The model under review builds one solid part; all positions refer to its coordinate system, in mm. A direction names the side the tool comes from. Coordinates: 2 decimals unless noted, no trailing zeros. Write each loop counter-clockwise with the first axis right and the second up, starting at its lowest first coordinate (ties: lowest second). Pieces come first, ordered by that corner, then holes. Notation, with made-up numbers: M 30.5,73 L 47.5,73 A24 cw 47.5,95 Z; hole C 34.5,17.5 d10. An arc over 180 degrees is marked long. Answer as CSV lines item,"result". Start each with the question number.
from build123d import *

# Parameters (mm, degrees)
BOSS_EXTRUDE1_DEPTH = 42
FILLET1_R           = 3
SKETCH3_R           = 4.25
CUT_EXTRUDE1_DEPTH  = 50.500549163
BOSS_EXTRUDE2_DEPTH = 42
CUT_EXTRUDE2_DEPTH  = 50.678098566


with BuildPart() as part:
    # Sketch1 → Boss-Extrude1 (new body)
    with BuildSketch(Plane(origin=(0, 0, 0), x_dir=(1, 0, 0), z_dir=(0, 1, 0))):
        with BuildLine():
            Line((-7.705313318, 23.08749092), (1.86118947, 26))
            ThreePointArc((1.86118947, 26), (5.698552556, 0), (1.86118947, -26))
            Line((1.86118947, -26), (-7.705313318, -23.08749092))
            ThreePointArc((-7.705313318, -23.08749092), (-4.301447444, 0), (-7.705313318, 23.08749092))
        make_face()
    extrude(amount=BOSS_EXTRUDE1_DEPTH)

    # Fillet1
    fillet1_edges = [part.edges().sort_by_distance(p)[0] for p in [
        (-7.705313318, 21, -23.08749092),
        (1.86118947, 21, -26),
        (1.86118947, 21, 26),
        (-7.705313318, 21, 23.08749092),
    ]]
    fillet(fillet1_edges, radius=FILLET1_R)

    # Sketch3 → Cut-Extrude1 (cut, through all)
    with BuildSketch(Plane(origin=(0, 42, 0), x_dir=(1, 0, 0), z_dir=(0, 1, 0))):
        with Locations(Location((0.733117745, 0, 0), (0, 0, 270))):
            Circle(SKETCH3_R)
    extrude(amount=-CUT_EXTRUDE1_DEPTH, mode=Mode.SUBTRACT)

    # Sketch4 → Boss-Extrude2 (add)
    with BuildSketch(Plane(origin=(0, 0, 0), x_dir=(1, 0, 0), z_dir=(0, 1, 0))):
        with BuildLine():
            Line((-3.757374772, -7.265548226), (-3.757374772, 7.265548226))
            ThreePointArc((-3.757374772, 7.265548226), (-8.179612228, 0), (-3.757374772, -7.265548226))
        make_face()
    extrude(amount=BOSS_EXTRUDE2_DEPTH)

    # Sketch5 → Cut-Extrude2 (cut, through all)
    with BuildSketch(Plane.XZ):
        with BuildLine():
            ThreePointArc((2.266407335, 16.5), (1.434288795, 18.123592589), (-0.36964556, 18.396163684))
            ThreePointArc((-0.36964556, 18.396163684), (0.266407335, 16.5), (0.832937896, 14.58191681))
            ThreePointArc((0.832937896, 14.58191681), (1.868446836, 15.302724159), (2.266407335, 16.5))
        make_face()
        with BuildLine():
            ThreePointArc((0.832937896, 14.58191681), (0.266407335, 16.5), (-0.36964556, 18.396163684))
            ThreePointArc((-0.36964556, 18.396163684), (-1.641032871, 15.898608399), (0.832937896, 14.58191681))
        make_face()
        with BuildLine():
            ThreePointArc((0.690987711, -15.08742552), (-1.795468684, -16.380384411), (-0.548037667, -18.889990746))
            ThreePointArc((-0.548037667, -18.889990746), (0.106129728, -17), (0.690987711, -15.08742552))
        make_face()
        with BuildLine():
            ThreePointArc((0.690987711, -15.08742552), (0.106129728, -17), (-0.548037667, -18.889990746))
            ThreePointArc((-0.548037667, -18.889990746), (1.266229984, -18.629161562), (2.106129728, -17))
            ThreePointArc((2.106129728, -17), (1.713879081, -15.810402582), (0.690987711, -15.08742552))
        make_face()
    extrude(amount=-CUT_EXTRUDE2_DEPTH, mode=Mode.SUBTRACT)


solid = part.part
1) To check wall thickness, follow line 1 (Z direction, x = 1.75, y = 18.5); line 2 (X direction, y = 20, z = -1.5); line 3 (X direction, y = 10, z = 15.5). State the ranges of each line that lie inside material, in increasing order. Write a range as [from, to].
2) Clearance check with flat-ended pins moving along their axes: pin 1 Ø8 at (x, z) = (1, -11) entering from -Y; pin 2 Ø3 at (y, z) = (36.5, -8) entering from +X; pin 3 Ø10 at (y, z) = (13, -18) entering from +X; pin 4 Ø3 at (y, z) = (33.5, 12.5) entering from +X. State where each tip first meets the part, or that it passes through.
3) Take a section at A-A on z = 0. Give the boundary of the cut face in (x, y).
4) Tool access review of faces 1 (the flat face through (-4, 42, 0)), 2 (the cylindrical face through (-5.45, 20.71, -13.5)): name each direction out of +Z, -Z, +X, -X, +Y, -Y from which nothing blocks a thin tool from reaching the whole face with its end or side.
5) Take a section at B-B on y = 26.5. Give the boundary of the cut face in (x, z), and give its area (3 significant figures).
6) Take a section at D-D on z = 10. Give the boundary of the cut face in (x, y).
7) Take a section at C-C on z = -16. Give the boundary of the cut face in (x, y), and give its area (3 significant figures).
8) Mouldability with a two-part tool opening along Z and no side actions: class faces 3 (the cylindrical face through (5.7, 20.7, -0.3)), 4 (the flat face through (-4, 0, 0)), 5 (the cylindrical face through (-5.48, 20.71, 13.69)), 6 (the cylindrical face through (-8.18, 20.71, -0.11)) as +Z half, -Z half, draft (parallel to the pull), parting line (faces both ways), or undercut.
Results:
1,line 1,"z = [-24.53, -18.14], [-15.86, -4.13], [4.13, 15.16], [17.84, 24.53]"
1,line 2,"x = [-8.04, -3.24], [4.71, 5.69]"
1,line 3,"x = [-5.82, -1.47], [2, 4.35]"
2,pin 1,"stops at y = 0"
2,pin 2,"stops at x = 5.46"
2,pin 3,"stops at x = 4.75"
2,pin 4,"stops at x = 5.02"
3,outline,"M -8.18,0 L -3.52,0 L -3.52,42 L -8.18,42 Z; M 4.98,0 L 5.7,0 L 5.7,42 L 4.98,42 Z"
4,face 1,"+Z, -Z, +X, -X, +Y"
4,face 2,"-X, +Y, -Y"
5,outline,"M -6.92,-20.31 A3 ccw -4.89,-23.94 L -1.07,-25.11 A3 ccw 2.71,-23.01 A90 ccw 2.71,23.01 A3 ccw -1.07,25.11 L -4.89,23.94 A3 ccw -6.92,20.31 A80 cw -4.59,6.77 A8.18 ccw -4.59,-6.77 A80 cw Z; hole C 0.73,0 d8.5; hole C 0.11,-17 d4; hole C 0.27,16.5 d4"
5,area,"445 mm²"
6,outline,"M -4.93,0 L 5.14,0 L 5.14,42 L -4.93,42 Z"
7,outline,"M -5.92,0 L -1.63,0 L -1.63,42 L -5.92,42 Z; M 1.84,0 L 4.26,0 L 4.26,42 L 1.84,42 Z"
7,area,"282 mm²"
8,face 3,"parting line"
8,face 4,"draft"
8,face 5,"undercut"
8,face 6,"undercut"
